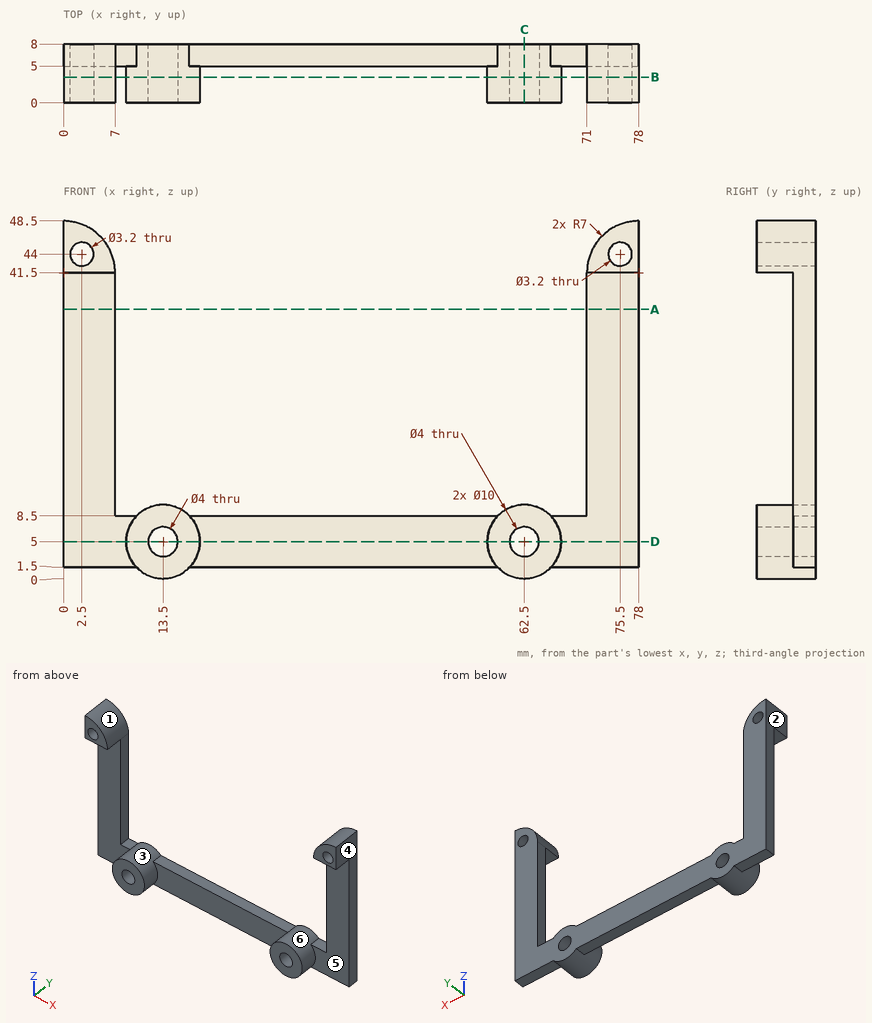
Drawing for the job (mm, zero at the part's lowest x, y, z). A direction names the side the tool comes from. Round coordinates to 2 decimals unless told otherwise and drop trailing zeros. Write each loop counter-clockwise with the first axis right and the second up, starting at its lowest first coordinate (ties: lowest second). Pieces come first, ordered by that corner, then holes. Notation, with made-up numbers: M 82.25,2.5 L 111.25,2.5 A30 ccw 111.25,35.5 Z; hole C -11.5,4.5 d4. An arc over 180 degrees is marked long. Put each result on its own line as item: value.
Item 1: Cut at A-A (z = 36.5). List the corners of the cut face in (x, y).
Responses:
outline: M 0,5 L 7,5 L 7,8 L 0,8 Z; M 71,5 L 78,5 L 78,8 L 71,8 Z
Item 2: Flat gauge pins, fed straight in: P1, Ø13, axis at x = 73, z = 15.5, coming from the -Y side; P2, Ø1.5, axis at x = 8, y = 7, coming from the +Z side; P3, Ø3.5, axis at x = 75.5, z = 44, coming from the -Y side; P4, Ø1.5, axis at x = 74.5, y = 6, coming from the -Z side. Where does each tip first touch, or does it go through?
Responses:
P1: y = 5
P2: z = 8.5
P3: y = 0
P4: z = 1.5
Item 3: Tool access for the marked faces 1, 2 and 3: list every direction of +Z, -Z, +X, -X, +Y, -Y with a clear straight run to the whole face (end or side of a thin tool).
Responses:
face 1: +Z, +Y, -Y
face 2: +Z, -Z, -X, +Y, -Y
face 3: -Y
Item 4: Mould opens along X. For the marked faces 4, 5 and 6 say: +X half, -X half, draft (parallel to the pull), parting line (faces both ways), or undercut.
Responses:
face 4: +X half
face 5: draft
face 6: undercut
Item 5: Cut at C-C (x = 62.5). List the corners of the cut face in (y, z), and give its area (3 significant figures).
Responses:
outline: M 0,0 L 8,0 L 8,3 L 0,3 Z; M 0,7 L 8,7 L 8,10 L 0,10 Z
area: 48.0 mm²
Item 6: Cut at D-D (z = 5). List the corners of the cut face in (x, y).
Responses:
outline: M 0,5 L 8.5,5 L 8.5,0 L 11.5,0 L 11.5,8 L 0,8 Z; M 15.5,0 L 18.5,0 L 18.5,5 L 57.5,5 L 57.5,0 L 60.5,0 L 60.5,8 L 15.5,8 Z; M 64.5,0 L 67.5,0 L 67.5,5 L 78,5 L 78,8 L 64.5,8 Z
Item 7: Probe L1, parallel to X at y = 6, z = 30.5; L2, parallel to X at y = 7, z = 45; L3, parallel to Y at x = 40.5, z = 4.5. List the from-to ranges inside material, lowest first. Write a range as from..to.
Responses:
L1: 0..7, 71..78
L2: 0..1.25, 3.75..6.06, 71.94..74.25, 76.75..78
L3: 5..8
Item 8: Cut at B-B (y = 3.5). List the corners of the cut face in (x, z).
Responses:
outline: M 0,41.5 L 7,41.5 A7 ccw 0,48.5 Z; C 13.5,5 d10; C 62.5,5 d10; M 71,41.5 L 78,41.5 L 78,48.5 A7 ccw Z; hole C 2.5,44 d3.2; hole C 13.5,5 d4; hole C 62.5,5 d4; hole C 75.5,44 d3.2
